from build123d import *

# Parameters (mm, degrees)
SKETCH1_W           = 164
SKETCH1_H           = 156
BOSS_EXTRUDE2_DEPTH = 87
SKETCH2_R           = 19.05
BOSS_EXTRUDE3_DEPTH = 87
BOSS_EXTRUDE3_DRAFT = -15
SHELL1_T            = -2.54


with BuildPart() as part:
    # Sketch1 → Boss-Extrude2 (new body)
    with BuildSketch(Plane(origin=(0, 0, 0), x_dir=(1, 0, 0), z_dir=(0, 1, 0))):
        Rectangle(SKETCH1_W, SKETCH1_H)
    extrude(amount=BOSS_EXTRUDE2_DEPTH)


with BuildPart() as boss_extrude3_tool:
    # Sketch2 → Boss-Extrude3 (with draft: the straight prism first)
    with BuildSketch(Plane(origin=(0, 87, 0), x_dir=(1, 0, 0), z_dir=(0, 1, 0))):
        Circle(SKETCH2_R)
    extrude(amount=BOSS_EXTRUDE3_DEPTH)
    # Boss-Extrude3: the draft: its side faces are tilted about the plane it starts from
    boss_extrude3_sides = [boss_extrude3_tool.faces().sort_by_distance(p)[0] for p in [
        (-19.05, 130.5, 0),
    ]]
    draft(boss_extrude3_sides, Plane(origin=(0, 87, 0), x_dir=(1, 0, 0), z_dir=(0, 1, 0)), BOSS_EXTRUDE3_DRAFT)


with BuildPart() as part_1:
    add(part.part)

    # Boss-Extrude3: add boss_extrude3_tool
    add(boss_extrude3_tool.part)

    # Shell1
    shell1_openings = [part_1.faces().sort_by_distance(p)[0] for p in [
        (0, 174, 0),
    ]]
    offset(amount=SHELL1_T, openings=shell1_openings, kind=Kind.INTERSECTION)


solid = part_1.part
Could you check a few things on this model? Use its own coordinates, in mm. A direction names the side the tool comes from. Round coordinates to 2 decimals unless told otherwise and drop trailing zeros. Order: outer loops, then holes, each group sorted by start corner. A loop starts at its lowest first (then second) coordinate and runs counter-clockwise, first axis right, second up. Notation, with made-up numbers: M -15.5,28.25 L 16.5,28.25 A21 cw 16.5,46.25 Z; hole C 57,75.25 d2. An arc over 180 degrees is marked long. One line per item, written item: value.
(1) Imagine slicing it at D-D (x = 0). Write out the boundary of the cut face in (y, z).
Ans:
outline: M 0,-78 L 87,-78 L 87,-19.05 L 174,-42.36 L 174,-39.73 L 84.46,-15.74 L 84.46,-75.46 L 2.54,-75.46 L 2.54,75.46 L 84.46,75.46 L 84.46,15.74 L 174,39.73 L 174,42.36 L 87,19.05 L 87,78 L 0,78 Z
(2) Imagine slicing it at C-C (z = 27.5). Count the separate pieces of the cut face and the enclosed holes in it, and give its area (3 significant figures).
Ans:
separate pieces: 2
enclosed holes: 1
area: 1,850 mm^2
(3) Imagine slicing it at A-A (y = 73.5). Write out the boundary of the cut face in (x, z), and give its area (3 significant figures).
Ans:
outline: M -82,-78 L 82,-78 L 82,78 L -82,78 Z; hole M -79.46,-75.46 L 79.46,-75.46 L 79.46,75.46 L -79.46,75.46 Z
area: 1,600 mm^2
(4) If we mould it in two halves opening along Y, with no side actions, what happens to faces 3 (the flat face through (-1, 43, -78)), 4 (the flat face through (-1, 2.54, -1)), 5 (the flat face through (-1, 0, -1)), 6 (the flat face through (-79.46, 43, 1))? For each: released by +Y, released by -Y, zero draft, split by the parting line, or undercut.
Ans:
face 3: zero draft
face 4: undercut
face 5: released by -Y
face 6: undercut
(5) I'm going to push a flat-ended pin straight in: P1, Ø6, axis at y = 97.5, z = -15.5, coming from the -X side. Where does the tip first touch, or does it pass through?
Ans:
P1: stops at x = -18.16
(6) Which directions (+Z, -Z, +X, -X, +Y, -Y) give clear straight access to the entire face, cutting with the end or side of a thin tool? Please do faces 1 (the conical face through (-6.06, 120.224, 27.288)), 2 (the flat face through (82, 43, 1)).
Ans:
face 1: none
face 2: +Z, -Z, +X, +Y, -Y
(7) I need wall thicknesses on line 1 along Y through (x, z) = (-45, 50.5); line 2 along Z through (x, y) = (37.5, 17); line 3 along X through (y, z) = (59, 54). Which ranges of each line are inside material? Lowest first, please. Write a range as from..to.
Ans:
line 1: y = 0..2.54, 84.46..87
line 2: z = -78..-75.46, 75.46..78
line 3: x = -82..-79.46, 79.46..82
(8) Imagine slicing it at B-B (z = 59.5). Write out the boundary of the cut face in (x, y).
Ans:
outline: M -82,0 L 82,0 L 82,87 L -82,87 Z; hole M -79.46,2.54 L 79.46,2.54 L 79.46,84.46 L -79.46,84.46 Z
